from build123d import *

# Parameters (mm, degrees)
SKETCH2_R           = 38.1
BOSS_EXTRUDE1_DEPTH = 4
SKETCH11_W          = 76.2
SKETCH11_H          = 77
BOSS_EXTRUDE4_DEPTH = 4
SKETCH3_R           = 0.8
CUT_EXTRUDE1_DEPTH  = 6
SKETCH4_R           = 0.6
CUT_EXTRUDE2_DEPTH  = 6
SKETCH5_W           = 1.5
SKETCH5_H           = 10
BOSS_EXTRUDE2_DEPTH = 10
CUT_EXTRUDE3_DEPTH  = 89.028915704
SKETCH7_R           = 1
CUT_EXTRUDE4_DEPTH  = 89.028915704
BOSS_EXTRUDE3_DEPTH = 8


with BuildPart() as part:
    # Sketch2 → Boss-Extrude1 (new body)
    with BuildSketch(Plane.XY):
        Circle(SKETCH2_R)
    extrude(amount=BOSS_EXTRUDE1_DEPTH)

    # Sketch11 → Boss-Extrude4 (add)
    with BuildSketch(Plane(origin=(0, 0, 0), x_dir=(-1, 0, 0), z_dir=(0, 0, -1))):
        with Locations((0, 38.5)):
            Rectangle(SKETCH11_W, SKETCH11_H)
    extrude(amount=-BOSS_EXTRUDE4_DEPTH)

    # Sketch3 → Cut-Extrude1 (cut)
    with BuildSketch(Plane.XY.offset(4)):
        with Locations((34.1, -0.085721815)):
            Circle(SKETCH3_R)
        with Locations((-17.05, -29.617188084)):
            Circle(SKETCH3_R)
        with Locations((-17.05, 29.445744454)):
            Circle(SKETCH3_R)
    extrude(amount=-CUT_EXTRUDE1_DEPTH, mode=Mode.SUBTRACT)

    # Sketch4 → Cut-Extrude2 (cut)
    with BuildSketch(Plane.XY.offset(4)):
        Circle(SKETCH4_R)
    extrude(amount=-CUT_EXTRUDE2_DEPTH, mode=Mode.SUBTRACT)

    # Sketch5 → Boss-Extrude2 (add)
    with BuildSketch(Plane.XY.offset(4)):
        with Locations((1.45, 0)):
            Rectangle(SKETCH5_W, SKETCH5_H)
        with Locations((-1.45, 0)):
            Rectangle(SKETCH5_W, SKETCH5_H)
    extrude(amount=BOSS_EXTRUDE2_DEPTH)

    # Sketch6 → Cut-Extrude3 (cut, through all)
    with BuildSketch(Plane(origin=(2.2, 0, 0), x_dir=(0, 0, -1), z_dir=(1, 0, 0))):
        with BuildLine():
            ThreePointArc((-14, 0), (-12.535533906, 3.535533906), (-9, 5))
            Line((-9, 5), (-14, 5))
            Line((-14, 5), (-14, 0))
        make_face()
        with BuildLine():
            ThreePointArc((-9, -5), (-12.535533906, -3.535533906), (-14, 0))
            Line((-14, 0), (-14, -5))
            Line((-14, -5), (-9, -5))
        make_face()
    extrude(amount=-CUT_EXTRUDE3_DEPTH, mode=Mode.SUBTRACT)

    # Sketch7 → Cut-Extrude4 (cut, through all)
    with BuildSketch(Plane(origin=(2.2, 0, 0), x_dir=(0, 0, -1), z_dir=(1, 0, 0))):
        with Locations(Location((-9, 2.3, 0), (0, 0, 90))):
            Circle(SKETCH7_R)
        with Locations(Location((-9, -2.8, 0), (0, 0, 90))):
            Circle(SKETCH7_R)
    extrude(amount=-CUT_EXTRUDE4_DEPTH, mode=Mode.SUBTRACT)

    # Sketch8 → Boss-Extrude3 (add)
    with BuildSketch(Plane.XY.offset(4)):
        Polygon((25.028792455, 0), (32.453413657, 7.424621202), (14.492901415, 25.385133445), (7.068280213, 17.960512242), align=None)
        Polygon((12.02011976, -15.101566346), (14.737719734, -25.243787522), (-9.796796254, -31.817791268), (-12.514396227, -21.675570092), align=None)
        Polygon((-19.088399973, -2.858945896), (-29.230621149, -0.141345922), (-22.656617403, 24.393170065), (-12.514396227, 21.675570092), align=None)
    extrude(amount=BOSS_EXTRUDE3_DEPTH)


solid = part.part
Could you check a few things on this model? Use its own coordinates, in mm. A direction names the side the tool comes from. Round coordinates to 2 decimals unless told otherwise and drop trailing zeros. Write each loop counter-clockwise with the first axis right and the second up, starting at its lowest first coordinate (ties: lowest second). Pieces come first, ordered by that corner, then holes. Notation, with made-up numbers: (79.25, 11) - (120.25, 11) arc R22 cw to (120.25, 47) - close; hole circle Ø5 at (78, 46.25). An arc over 180 degrees is marked (long way). Use a Markdown table: item, result.
Q1. Thinking about a two-plate mould opening in X: for faces 1 (the flat face through (20, 13, 12)), 2 (the flat face through (0.7, 0, 9)), 3 (the flat face through (23.6, 16.28, 7.94)), which applies, released by +X, released by -X, zero draft, split by the parting line, or undercut?
Output values:
| item | result |
|---|---|
| face 1 | zero draft |
| face 2 | undercut |
| face 3 | released by +X |
Q2. I want a section at C-C (y = 52). List the corners of the cut face in (x, z) for me, plus the area to 3 significant figures.
Output values:
| item | result |
|---|---|
| outline | (-38.1, 0) - (38.1, 0) - (38.1, 4) - (-38.1, 4) - close |
| area | 305 mm2 |
Q3. Please list where these lines run through material, in increasing order: L1, parallel to Y at x = -17.05, z = 1.7; L2, parallel to Z at x = -10, y = -21.5; L3, parallel to Z at x = -1.25, y = 2.3.
Output values:
| item | result |
|---|---|
| L1 | -34.07 to -30.42, -28.82 to 28.65, 30.25 to 77 |
| L2 | 0 to 12 |
| L3 | 0 to 8, 10 to 13.44 |
Q4. For faces 4 (the flat face through (1, 20, 4)), 5 (the flat face through (28.69, 3.66, 7.94)), 6 (the flat face through (13.36, -20.1, 7.94)), 7 (the flat face through (-0.7, 0, 9)), which set-ups out of +Z, -Z, +X, -X, +Y, -Y let a thin tool reach every point of the face, with its end or its side?
Output values:
| item | result |
|---|---|
| face 4 | +Z |
| face 5 | +Z, +X, -Y |
| face 6 | +Z, +X |
| face 7 | +Z, +Y |
Q5. I want a section at B-B (x = 21). List the corners of the cut face in (y, z) for me, plus the area to 3 significant figures.
Output values:
| item | result |
|---|---|
| outline | (-31.79, 0) - (77, 0) - (77, 4) - (18.88, 4) - (18.88, 12) - (4.03, 12) - (4.03, 4) - (-31.79, 4) - close |
| area | 554 mm2 |
Q6. I want a section at A-A (z = 1.75). List the corners of the cut face in (x, y) for me, plus the area to 3 significant figures.
Output values:
| item | result |
|---|---|
| outline | (-38.1, 0) arc R38.1 ccw to (38.1, 0) - (38.1, 77) - (-38.1, 77) - close; hole circle Ø1.6 at (-17.05, -29.62); hole circle Ø1.6 at (-17.05, 29.45); hole circle Ø1.2 at (0, 0); hole circle Ø1.6 at (34.1, -0.09) |
| area | 8,140 mm2 |
Q7. I want a section at D-D (x = -26.5). List the corners of the cut face in (y, z) for me, plus the area to 3 significant figures.
Output values:
| item | result |
|---|---|
| outline | (-27.37, 0) - (77, 0) - (77, 4) - (10.05, 4) - (10.05, 12) - (-0.87, 12) - (-0.87, 4) - (-27.37, 4) - close |
| area | 505 mm2 |
Q8. For pin 1 (1.2 mm diameter, centred on x = 2, z = 6, fed in from +Y); pin 2 (4 mm diameter, centred on x = -9.5, y = 20.5, fed in from +Z); pin 3 (3 mm diameter, centred on y = 14, z = 11, fed in from +X), each with a flat end and sliding along its axis, tell me the tip position at first contact or that it passes through.
Output values:
| item | result |
|---|---|
| pin 1 | y = 5 |
| pin 2 | z = 4 |
| pin 3 | x = 27.38 |
